Verification items for the finished model (mm, model axes). A direction names the side the tool comes from. Coordinates: 2 decimals unless noted, no trailing zeros. Write each loop counter-clockwise with the first axis right and the second up, starting at its lowest first coordinate (ties: lowest second). Pieces come first, ordered by that corner, then holes. Notation, with made-up numbers: (62.5, 52) -> (97.5, 52) arc R35 cw to (97.5, 90) -> close; hole circle Ø11 at (62, 88.5). An arc over 180 degrees is marked (long way). Answer in a Markdown table with one row per item.
```python
from build123d import *

# Parameters (mm, degrees)
F0_R     = 25
F1_DEPTH = 3
F0_R_2   = 30
F2_DEPTH = 5
F4_R     = 2.5019013152
F5_DEPTH = 25


# Not quite as in the source:
# - a fillet or chamfer that OpenCascade refuses, or shapes differently, is made with other operations: its cross-section is extruded or revolved along the edge and cut away or added


with BuildPart() as f1:
    # F0 (on Top) → F1 (new body)
    with BuildSketch(Plane.XY):
        Circle(F0_R)
    extrude(amount=F1_DEPTH)

    # F0 (on Top) → F2 (join)
    with BuildSketch(Plane.XY):
        Circle(F0_R_2)
        Circle(F0_R, mode=Mode.SUBTRACT)
    extrude(amount=F2_DEPTH)

    # F3: fillet of radius 2.5 on 2 edges, made by hand

    # F3_s1 → F3_t2 (revolve, cut)
    with BuildSketch(Plane.XZ):
        with BuildLine():
            ThreePointArc((30, 2.5), (29.267766953, 4.267766953), (27.5, 5))
            Line((27.5, 5), (30, 5))
            Line((30, 5), (30, 2.5))
        make_face()
    revolve(axis=Axis((0, 0, 5), (0, 0, 1)), mode=Mode.SUBTRACT)

    # F3_s3 → F3_t4 (revolve, cut)
    with BuildSketch(Plane.XZ):
        with BuildLine():
            ThreePointArc((27.4494897428, 5), (25.8683509127, 4.4364916731), (25, 3))
            Line((25, 3), (25, 5))
            Line((25, 5), (27.4494897428, 5))
        make_face()
    revolve(axis=Axis((0, 0, 5), (0, 0, 1)), mode=Mode.SUBTRACT)

    # F4 (on face) → F5 (cut)
    with BuildSketch(Plane.XY.offset(3)):
        with Locations((-7.9056667164, 8.0453660339)):
            Circle(F4_R)
        with Locations((7.9056667164, -8.0453660339)):
            Circle(F4_R)
        with Locations((7.9056667164, 8.0453660339)):
            Circle(F4_R)
        with Locations((-7.9056667164, -8.0453660339)):
            Circle(F4_R)
    extrude(amount=-F5_DEPTH, mode=Mode.SUBTRACT)


solid = f1.part
```
1. Section check A-A, the plane y = 0. Record the boundary of the cut face in (x, z), plus the area to 3 significant figures.
Geometry says:
| item | result |
|---|---|
| outline | (-30, 0) -> (30, 0) -> (30, 2.5) arc R2.5 ccw to (27.5, 5) -> (27.45, 5) arc R2.5 ccw to (25, 3) -> (-25, 3) arc R2.5 ccw to (-27.45, 5) -> (-27.5, 5) arc R2.5 ccw to (-30, 2.5) -> close |
| area | 195 mm^2 |
2. Mould release check, pull along X, two halves, no side actions. Record for faces 3 (the flat face through (0, 0, 0)), 4 (the cylindrical face through (-10.405, -7.935, 1.521)), 5 (the cylindrical face through (-29.97, 1.32, 1.23)): released by +X, released by -X, zero draft, split by the parting line, or undercut.
Geometry says:
| item | result |
|---|---|
| face 3 | zero draft |
| face 4 | undercut |
| face 5 | split by the parting line |
3. Section check D-D, the plane y = -9.5. State how many separate pieces and enclosed holes the cut face has, plus the area to 3 significant figures.
Geometry says:
| item | result |
|---|---|
| separate pieces | 3 |
| enclosed holes | 0 |
| area | 162 mm^2 |
4. Thickness scan on line 1 (X direction, y = -7, z = 0.8); line 2 (Y direction, x = -10, z = 2.4); line 3 (Y direction, x = -12, z = 2.45). Record the ranges inside material, lowest first. Write a range as from..to.
Geometry says:
| item | result |
|---|---|
| line 1 | -29.17..-10.18, -5.63..5.63, 10.18..29.17 |
| line 2 | -28.28..-9.41, -6.68..6.68, 9.41..28.28 |
| line 3 | -27.5..27.5 |
5. Section check C-C, the plane z = 1.2. Record the boundary of the cut face in (x, y), plus the area to 3 significant figures.
Geometry says:
| item | result |
|---|---|
| outline | circle Ø60 at (0, 0); hole circle Ø5 at (-7.91, -8.05); hole circle Ø5 at (-7.91, 8.05); hole circle Ø5 at (7.91, -8.05); hole circle Ø5 at (7.91, 8.05) |
| area | 2,750 mm^2 |
6. Depth check by flat-ended pin: P1, Ø2, axis at y = -20, z = 1.5, coming from the -X side; P2, Ø2, axis at x = 2, z = 2.5, coming from the +Y side; P3, Ø3, axis at y = 19, z = 2, coming from the -X side. Enter the tip coordinate at first touch or a pass-through.
Geometry says:
| item | result |
|---|---|
| P1 | x = -23.22 |
| P2 | y = 29.98 |
| P3 | x = -24.37 |
7. Tool access check on faces 1 (the flat face through (0, 0, 3)), 2 (the cylindrical face through (10.22, 7.09, 1.52)). Record the directions out of +Z, -Z, +X, -X, +Y, -Y that give a thin tool (end or side, any length) a straight path to the whole face; none if there is none.
Geometry says:
| item | result |
|---|---|
| face 1 | +Z |
| face 2 | +Z, -Z |
